from build123d import *

# Parameters (mm, degrees)
BOSS_EXTRUDE1_DEPTH = 3


with BuildPart() as part:
    # Sketch2 → Boss-Extrude1 (new body, symmetric)
    with BuildSketch(Plane.ZY.offset(34.45)):
        with BuildLine():
            Line((-38.720907523, 77.254093909), (41.048520471, 63.188591518))
            ThreePointArc((41.048520471, 63.188591518), (47.023521903, 54.655405132), (38.490335517, 48.6804037))
            Line((38.490335517, 48.6804037), (-41.279092477, 62.745906091))
            ThreePointArc((-41.279092477, 62.745906091), (-47.254093909, 71.279092477), (-38.720907523, 77.254093909))
        make_face()
        with BuildLine():
            Line((-38.98137979, 75.776882279), (40.788048204, 61.711379888))
            ThreePointArc((40.788048204, 61.711379888), (45.546310273, 54.915877399), (38.750807784, 50.15761533))
            Line((38.750807784, 50.15761533), (-41.01862021, 64.223117721))
            ThreePointArc((-41.01862021, 64.223117721), (-45.776882279, 71.01862021), (-38.98137979, 75.776882279))
        make_face(mode=Mode.SUBTRACT)
    extrude(amount=BOSS_EXTRUDE1_DEPTH, both=True)


solid = part.part
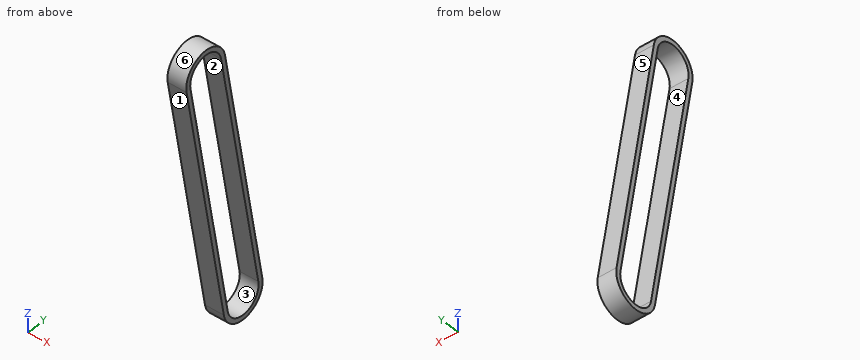
CAD build for the part. Positions are in the model's coordinates, mm. Face numbers are marked on the shaded views. A direction names the side the tool comes from. Round coordinates to 2 decimals unless told otherwise and drop trailing zeros. Write each loop counter-clockwise with the first axis right and the second up, starting at its lowest first coordinate (ties: lowest second). Pieces come first, ordered by that corner, then holes. Notation, with made-up numbers: (10, 76) -> (49, 76) arc R14 cw to (49, 103) -> close; hole circle Ø2 at (30.5, -3). An arc over 180 degrees is marked (long way). Answer as a JSON object with one key per item and string values.
(1) Band-saw the part on B-B, the plane x = -33.9. List the corners of the cut face in (y, z), then the cut area to 3 significant figures.
Reported:
{"outline": "(48.68, 38.49) -> (62.75, -41.28) arc R7.37 ccw to (77.25, -38.72) -> (63.19, 41.05) arc R7.37 ccw to start; hole (50.16, 38.75) -> (64.22, -41.02) arc R5.87 ccw to (75.78, -38.98) -> (61.71, 40.79) arc R5.87 ccw to start", "area": "305 mm^2"}
(2) Two-plate mould, pull along Y, no slides. Class the marked faces 3, 4, 5 and 6: +Y half, -Y half, draft (parallel to the pull), parting line (faces both ways), or undercut.
Reported:
{"face 3": "undercut", "face 4": "undercut", "face 5": "+Y half", "face 6": "parting line"}
(3) Band-saw the part on A-A, the plane z = -40. List the corners of the cut face in (x, y), then the cut area to 3 significant figures.
Reported:
{"outline": "(-37.45, 62.52) -> (-31.45, 62.52) -> (-31.45, 64.04) -> (-37.45, 64.04) -> close; (-37.45, 75.87) -> (-31.45, 75.87) -> (-31.45, 77.37) -> (-37.45, 77.37) -> close", "area": "18.1 mm^2"}
(4) Band-saw the part on C-C, the plane y = 70.75. List the corners of the cut face in (x, z), then the cut area to 3 significant figures.
Reported:
{"outline": "(-37.45, -47.33) -> (-31.45, -47.33) -> (-31.45, -45.82) -> (-37.45, -45.82) -> close; (-37.45, -10.47) -> (-31.45, -10.47) -> (-31.45, -1.83) -> (-37.45, -1.83) -> close", "area": "60.9 mm^2"}
(5) Pin check, flat tips, straight feed: P1, Ø5, axis at y = 59.5, z = 30.5, coming from the +X side (3 decimals); P2, Ø1, axis at x = -33.5, z = -12.5, coming from the +Y side. Stop position of each tip, or through.
Reported:
{"P1": "passes through", "P2": "stops at y = 72.72"}
(6) Probe probe 1 along Y at (x, z) = (-34.5, 0.5); probe 2 along Y at (x, z) = (-32, -8.5). List the from-to ranges inside material, lowest first. Write a range as [from, to].
Reported:
{"probe 1": "y = [55.38, 56.9], [68.82, 70.34]", "probe 2": "y = [56.97, 58.49], [70.4, 71.93]"}
(7) Which spindle directions (+Z, -Z, +X, -X, +Y, -Y) get a long thin tool onto all of the face, cutting with end or side? Do the marked faces 1 and 2. Say none if no direction does.
Reported:
{"face 1": "-Z, +X, -X, -Y", "face 2": "+X, -X"}
